Check sheet for the drawn part. Datum: minimum x, y, z corner. Units: mm. A direction names the side the tool comes from. Round coordinates to 2 decimals unless told otherwise and drop trailing zeros. Order: outer loops, then holes, each group sorted by start corner. A loop starts at its lowest first (then second) coordinate and runs counter-clockwise, first axis right, second up. Notation, with made-up numbers: (65, 34) - (104, 34) arc R23 cw to (104, 70) - close; hole circle Ø11 at (-10.75, 46). An arc over 180 degrees is marked (long way). Write each question's results on one line, items separated by ' | '.
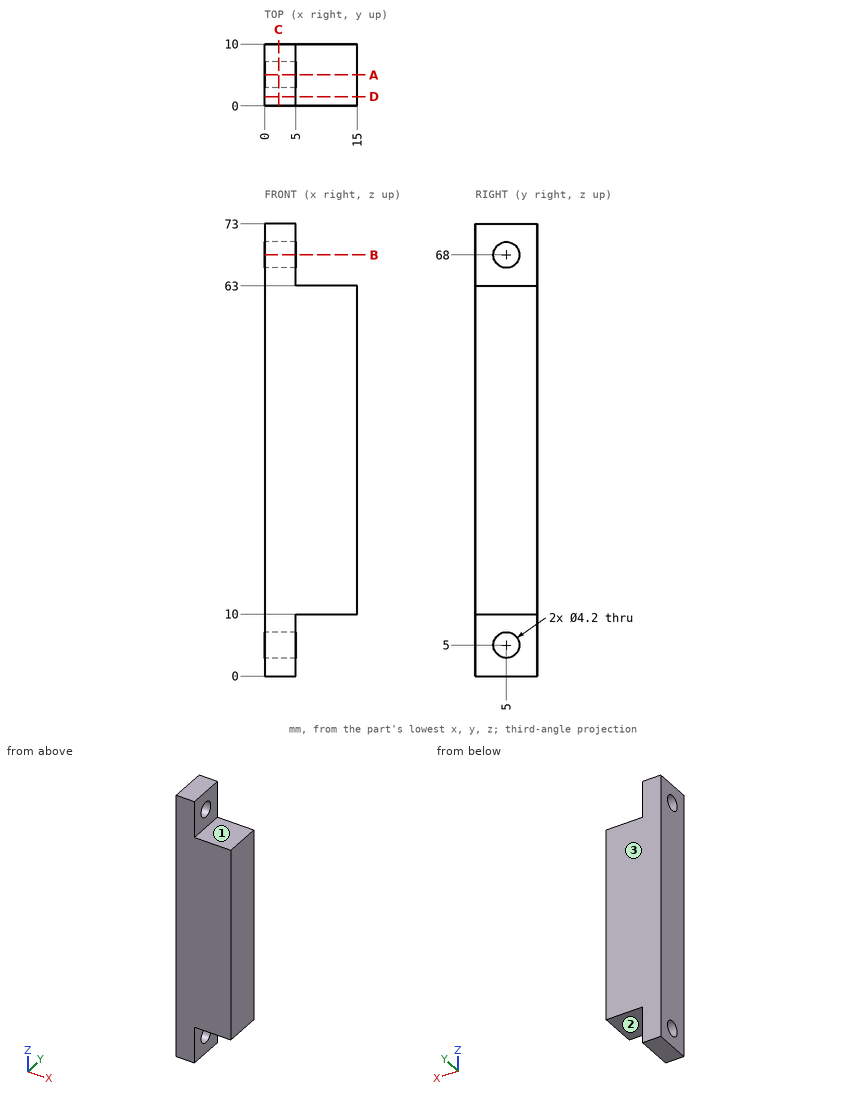
(1) Section check B-B (z = 68). Record the cut outline in (x, y).
Answers follow:
outline: (0, 0) - (5, 0) - (5, 2.9) - (0, 2.9) - close; (0, 7.1) - (5, 7.1) - (5, 10) - (0, 10) - close
(2) Access from +Z, -Z, +X, -X, +Y, -Y to the whole of each face (thin tool, end or side, straight path). Record for the marked faces 1, 2 and 3.
Answers follow:
face 1: +Z, +X, +Y, -Y | face 2: -Z, +X, +Y, -Y | face 3: +Z, -Z, +X, -X, +Y
(3) Depth check by flat-ended pin: pin 1 Ø3.5 at (y, z) = (5, 68) entering from -X; pin 2 Ø5 at (x, y) = (9.5, 6.5) entering from -Z; pin 3 Ø3 at (x, y) = (12, 4) entering from +Z; pin 4 Ø3 at (y, z) = (3.5, 66.5) entering from +X. Enter the tip coordinate at first touch or a pass-through.
Answers follow:
pin 1: through | pin 2: z = 10 | pin 3: z = 63 | pin 4: x = 5
(4) Section check A-A (y = 5). Record the cut outline in (x, z), then the cut area to 3 significant figures.
Answers follow:
outline: (0, 0) - (5, 0) - (5, 2.9) - (0, 2.9) - close; (0, 7.1) - (5, 7.1) - (5, 10) - (15, 10) - (15, 63) - (5, 63) - (5, 65.9) - (0, 65.9) - close; (0, 70.1) - (5, 70.1) - (5, 73) - (0, 73) - close | area: 853 mm²
(5) Section check D-D (y = 1.5). Record the cut outline in (x, z).
Answers follow:
outline: (0, 0) - (5, 0) - (5, 10) - (15, 10) - (15, 63) - (5, 63) - (5, 73) - (0, 73) - close
(6) Material ranges on line 1 (Z direction, x = 2.65, y = 5); line 2 (Y direction, x = 3.95, z = 68); line 3 (Z direction, x = 2.75, y = 3.5), recorded low to high.
Answers follow:
line 1: 0 to 2.9, 7.1 to 65.9, 70.1 to 73 | line 2: 0 to 2.9, 7.1 to 10 | line 3: 0 to 3.53, 6.47 to 66.53, 69.47 to 73
(7) Section check C-C (x = 2.25). Record the cut outline in (y, z).
Answers follow:
outline: (0, 0) - (10, 0) - (10, 73) - (0, 73) - close; hole circle Ø4.2 at (5, 5); hole circle Ø4.2 at (5, 68)
